Input: dimensioned drawing with shaded views. Units: mm. Origin: part minimum x, y, z. Give positions to 0.01 mm unless a question says otherwise; leave off trailing zeros. Loops run counter-clockwise (first coordinate to the right, second up) from the corner with the lowest first, then second, coordinate; pieces in that order, holes last. Notation, with made-up numbers: (-18, 60) -> (-12, 60) arc R24 ccw to (-12, 81) -> close; hole circle Ø6 at (74, 38.25). An arc over 180 degrees is marked (long way). Answer as a JSON object with one key per item and string values.
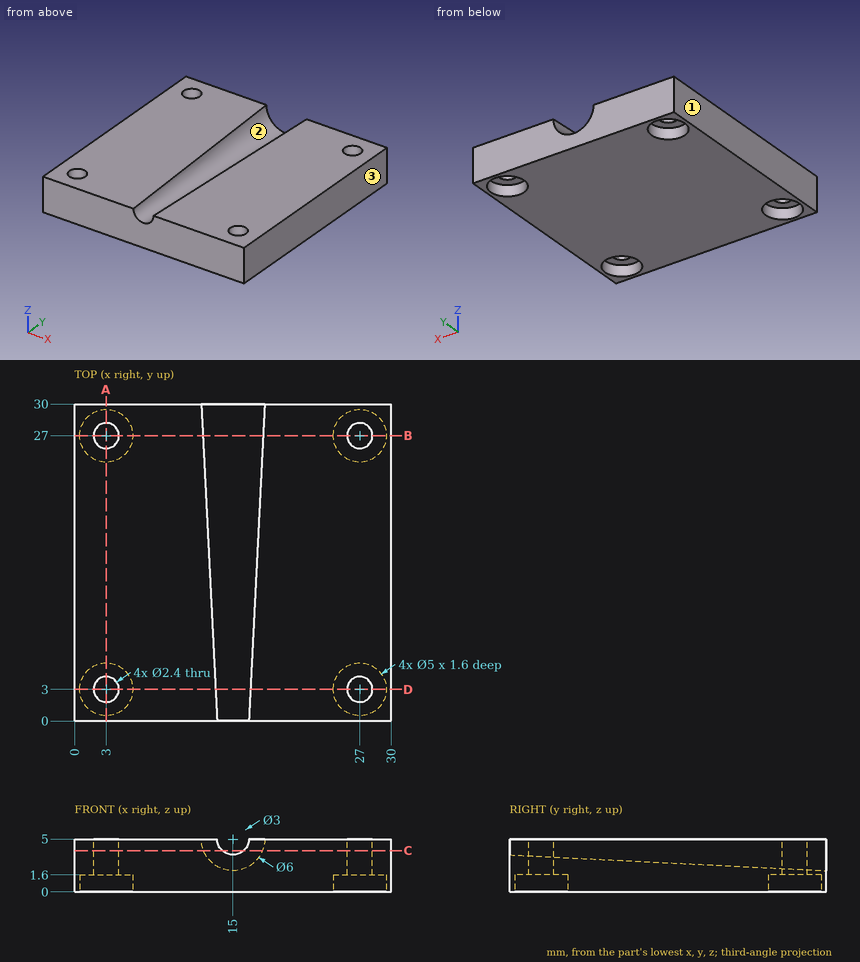
Q1. Section A-A, the plane x = 3. Return the cut outline in (y, z), then the cut area to 3 significant figures.
Evaluation:
{"outline": "(0, 0) -> (0.5, 0) -> (0.5, 1.6) -> (1.8, 1.6) -> (1.8, 5) -> (0, 5) -> close; (4.2, 1.6) -> (5.5, 1.6) -> (5.5, 0) -> (24.5, 0) -> (24.5, 1.6) -> (25.8, 1.6) -> (25.8, 5) -> (4.2, 5) -> close; (28.2, 1.6) -> (29.5, 1.6) -> (29.5, 0) -> (30, 0) -> (30, 5) -> (28.2, 5) -> close", "area": "118 mm2"}
Q2. Section D-D, the plane y = 3. Return the cut outline in (x, z).
Evaluation:
{"outline": "(0, 0) -> (0.5, 0) -> (0.5, 1.6) -> (1.8, 1.6) -> (1.8, 5) -> (0, 5) -> close; (4.2, 1.6) -> (5.5, 1.6) -> (5.5, 0) -> (24.5, 0) -> (24.5, 1.6) -> (25.8, 1.6) -> (25.8, 5) -> (16.65, 5) arc R1.65 cw to (13.35, 5) -> (4.2, 5) -> close; (28.2, 1.6) -> (29.5, 1.6) -> (29.5, 0) -> (30, 0) -> (30, 5) -> (28.2, 5) -> close"}
Q3. Section B-B, the plane y = 27. Return the cut outline in (x, z).
Evaluation:
{"outline": "(0, 0) -> (0.5, 0) -> (0.5, 1.6) -> (1.8, 1.6) -> (1.8, 5) -> (0, 5) -> close; (4.2, 1.6) -> (5.5, 1.6) -> (5.5, 0) -> (24.5, 0) -> (24.5, 1.6) -> (25.8, 1.6) -> (25.8, 5) -> (17.85, 5) arc R2.85 cw to (12.15, 5) -> (4.2, 5) -> close; (28.2, 1.6) -> (29.5, 1.6) -> (29.5, 0) -> (30, 0) -> (30, 5) -> (28.2, 5) -> close"}
Q4. Ray query, line 1 along Y through (x, z) = (3, 0.9); line 2 along Y through (x, z) = (27, 3.85); line 3 along X through (y, z) = (11, 3.6). Return the intervals inside material, ascending.
Evaluation:
{"line 1": "y = 0 to 0.5, 5.5 to 24.5, 29.5 to 30", "line 2": "y = 0 to 1.8, 4.2 to 25.8, 28.2 to 30", "line 3": "x = 0 to 13.5, 16.5 to 30"}
Q5. Pin query (flat end, axial travel): pin 1 (1.5 mm diameter, centred on x = 26, y = 27, fed in from -Z). Return the tip coordinate at first contact, or that it passes through.
Evaluation:
{"pin 1": "stops at z = 1.6"}
Q6. Section C-C, the plane z = 3.9. Give the number of separate pieces and of enclosed holes in the cut face, then the cut area to 3 significant figures.
Evaluation:
{"separate pieces": "2", "enclosed holes": "4", "area": "765 mm2"}
Q7. Draft query along X for the marked faces 1, 2 and 3. Return one class per face: +X half, -X half, draft (parallel to the pull), parting line (faces both ways), or undercut.
Evaluation:
{"face 1": "-X half", "face 2": "undercut", "face 3": "+X half"}
